For this review, take the finished solid that the model builds, in its own axes (mm). A direction names the side the tool comes from. Give positions to 0.01 mm unless a question says otherwise; leave off trailing zeros. Order: outer loops, then holes, each group sorted by start corner. A loop starts at its lowest first (then second) coordinate and runs counter-clockwise, first axis right, second up.
Item 1: For P1, Ø1, axis at x = 21.5, z = -137, coming from the +Y side; P2, Ø5, axis at x = 24, z = -85.5, coming from the -Y side; P3, Ø12, axis at x = 68.5, z = -72.5, coming from the -Y side; P4, Ø9.5, axis at x = 95.5, z = -73.5, coming from the +Y side, all flat-tipped, find the tip position at first contact; note any pin that passes through.
Item 2: Consider section B-B (z = -130). Give the boundary of the cut face in (x, y), plus the area to 3 significant figures.
Item 3: Consider section D-D (x = 92.5). Give the boundary of the cut face in (y, z), plus the area to 3 significant figures.
Item 4: Consider section A-A (x = 28). Give the boundary of the cut face in (y, z).
Item 5: Consider section C-C (y = 21). Give the boundary of the cut face in (x, z).
Item 6: For probe 1 along Y at (x, z) = (34.5, -130); probe 2 along Y at (x, z) = (44, -70); probe 3 along X at (y, z) = (52.5, -146), list the stretches that pass through material, from the lowest coordinate up.
Item 7: Machinability: for faces 5 (the cylindrical face through (50.532, 95.993, -129.34)), 6 (the flat face through (50, 10, -79)), 7 (the flat face through (94, 12, -79)), 8 (the flat face through (75, 24, -49)), which of the approach directions +Z, -Z, +X, -X, +Y, -Y give a long, thin tool a straight path to every point of the face, cutting with its end or side? Answer none if there is none.
Item 8: The part is to be moulded in two halves that separate along X. For faces 1 (the flat face through (31, 24, -49)), 2 (the flat face through (62, 46, -64)), 3 (the flat face through (24, 5, -79)), 4 (the flat face through (76, 5, -79)), say which applies: released by +X, released by -X, zero draft, split by the parting line, or undercut.
```python
from build123d import *

# Parameters (mm, degrees)
BOSS_EXTRUDE1_DEPTH = 160
SKETCH3_R           = 15
BOSS_EXTRUDE3_DEPTH = 76
RIB2_REACH          = 196.813
SKETCH5_WALL_W      = 524.907117832
SKETCH5_WALL_H      = 12


with BuildPart() as part:
    # Sketch2 → Boss-Extrude1 (new body)
    with BuildSketch(Plane.XY):
        Polygon((0, 0), (0, 12), (12, 12), (12, 24), (88, 24), (88, 12), (100, 12), (100, 0), (76, 0), (76, 10), (24, 10), (24, 0), align=None)
    extrude(amount=-BOSS_EXTRUDE1_DEPTH)

    # Sketch3 → Boss-Extrude3 (add)
    with BuildSketch(Plane(origin=(88, 0, 0), x_dir=(0, 0, -1), z_dir=(1, 0, 0))):
        with BuildLine():
            Line((100, 24), (100, 66))
            ThreePointArc((100, 66), (130, 96), (160, 66))
            Line((160, 66), (160, 24))
            Line((160, 24), (100, 24))
        make_face()
        with Locations((130, 66)):
            Circle(SKETCH3_R, mode=Mode.SUBTRACT)
    extrude(amount=-BOSS_EXTRUDE3_DEPTH)

    # Sketch5 wall → Rib2 (add, up to next)
    with BuildSketch(Plane(origin=(56, 57.912517706, -57.366725049), x_dir=(0, 0.508884996756, -0.860834513758), z_dir=(0, 0.860834513758, 0.508884996756)), mode=Mode.PRIVATE) as rib2_sk1:
        Rectangle(SKETCH5_WALL_W, SKETCH5_WALL_H)
    rib2_tool1 = extrude(rib2_sk1.sketch, amount=-RIB2_REACH, mode=Mode.PRIVATE) - part.part
    add(rib2_tool1.solids().sort_by_distance((56, 57.912517706, -57.366725049))[0])


solid = part.part
```
Resolved:
1. P1: stops at y = 95.29
1. P2: stops at y = 0
1. P3: stops at y = 10
1. P4: stops at y = 12
2. outline: (0, 0) - (24, 0) - (24, 10) - (76, 10) - (76, 0) - (100, 0) - (100, 12) - (88, 12) - (88, 51) - (12, 51) - (12, 12) - (0, 12) - close; (12, 81) - (88, 81) - (88, 96) - (12, 96) - close
2. area: 4,780 mm2
3. outline: (0, -160) - (12, -160) - (12, 0) - (0, 0) - close
3. area: 1,920 mm2
4. outline: (10, -160) - (66, -160) arc R30 ccw to (66, -100) - (24, -100) - (24, 0) - (10, 0) - close; hole circle Ø30 at (66, -130)
5. outline: (12, -160) - (88, -160) - (88, 0) - (12, 0) - close
6. probe 1: y = 10 to 51, 81 to 96
6. probe 2: y = 10 to 24
6. probe 3: x = 12 to 88
7. face 5: +Y
7. face 6: +Z, -Z, -Y
7. face 7: +Z, -Z, +X, +Y
7. face 8: +Z, +X, +Y
8. face 1: zero draft
8. face 2: released by +X
8. face 3: undercut
8. face 4: undercut
